from build123d import *

# Parameters (mm, degrees)
DOME_TRIM_SKETCH_W           = 13.999999999999993
DOME_TRIM_SKETCH_H           = 5.000000000000014
DOME_TRIM_DEPTH              = 14
RETAINER_FEATURE_3_PROFILE_R = 3.0000000000000027
RETAINER_FEATURE_3_DEPTH     = 3
RETAINER_FEATURE_4_PROFILE_R = 3.0000000000000027
RETAINER_FEATURE_4_DEPTH     = 3
RETAINER_FEATURE_6_PROFILE_R = 1.1000000000000036
RETAINER_FEATURE_6_DEPTH     = 4.25
RETAINER_FEATURE_7_PROFILE_R = 2.1000000000000045
RETAINER_FEATURE_7_DEPTH     = 1.45
RETAINER_FEATURE_8_PROFILE_R = 1.1000000000000036
RETAINER_FEATURE_8_DEPTH     = 4.25
RETAINER_FEATURE_9_PROFILE_R = 2.1000000000000045
RETAINER_FEATURE_9_DEPTH     = 1.45
RETAINER_FEATURE_12_DEPTH    = 10


with BuildPart() as part:
    # Retainer Dome Sketch → Retainer Dome (revolve)
    with BuildSketch(Plane(origin=(0, -73, 0), x_dir=(-1, 0, 0), z_dir=(0, -1, 0))):
        with BuildLine():
            Line((76.48780366869515, -22.98076211353316), (66.09549882328189, -28.980762113533164))
            ThreePointArc((66.09549882328189, -28.980762113533164), (74.29165124598852, -31.176914536239792), (76.48780366869515, -22.98076211353316))
        make_face()
    revolve(axis=Axis((-62.63139720814413, -73, 30.98076211353316), (-0.8660254037844387, 0, -0.49999999999999994)))

    # Dome Trim Sketch → Dome Trim (cut)
    with BuildSketch(Plane(origin=(-36.156560608000376, 0, -20.874999999999996), x_dir=(-0.49999999999999944, 0, 0.866025403784439), z_dir=(-0.866025403784439, 0, -0.49999999999999944))):
        with Locations((58.145825622994224, -68.5)):
            Rectangle(DOME_TRIM_SKETCH_W, DOME_TRIM_SKETCH_H)
    extrude(amount=DOME_TRIM_DEPTH, mode=Mode.SUBTRACT)

    # Retainer Feature 3 profile → Retainer Feature 3 (add)
    with BuildSketch(Plane(origin=(0, -71.00000000000001, 0), x_dir=(-1, 0, 0), z_dir=(0, -1, 0))):
        with Locations((63.93043531382078, -30.23076211353316)):
            Circle(RETAINER_FEATURE_3_PROFILE_R)
    extrude(amount=RETAINER_FEATURE_3_DEPTH)

    # Retainer Feature 4 profile → Retainer Feature 4 (add)
    with BuildSketch(Plane(origin=(0, -71.00000000000001, 0), x_dir=(-1, 0, 0), z_dir=(0, -1, 0))):
        with Locations((78.65286717815624, -21.73076211353316)):
            Circle(RETAINER_FEATURE_4_PROFILE_R)
    extrude(amount=RETAINER_FEATURE_4_DEPTH)

    # Spherical Seat Sketch → Spherical Seat (revolve, cut)
    with BuildSketch(Plane(origin=(0, -73, 0), x_dir=(-1, 0, 0), z_dir=(0, -1, 0))):
        with BuildLine():
            Line((74.0196312679095, -24.405762113533164), (68.56367122406753, -27.55576211353316))
            ThreePointArc((68.56367122406753, -27.55576211353316), (72.86665124598852, -28.708742135454145), (74.0196312679095, -24.405762113533164))
        make_face()
    revolve(axis=Axis((-62.63139720814413, -73, 30.98076211353316), (-0.8660254037844387, 0, -0.49999999999999994)), mode=Mode.SUBTRACT)

    # Retainer Feature 6 profile → Retainer Feature 6 (cut)
    with BuildSketch(Plane(origin=(0, -70, 0), x_dir=(-1, 0, 0), z_dir=(0, -1, 0))):
        with Locations(Location((63.93043531382078, -30.23076211353316, 0), (0, 0, 270))):
            Circle(RETAINER_FEATURE_6_PROFILE_R)
    extrude(amount=RETAINER_FEATURE_6_DEPTH, mode=Mode.SUBTRACT)

    # Retainer Feature 7 profile → Retainer Feature 7 (cut)
    with BuildSketch(Plane(origin=(0, -72.8, 0), x_dir=(-1, 0, 0), z_dir=(0, -1, 0))):
        with Locations(Location((63.93043531382078, -30.23076211353316, 0), (0, 0, 90))):
            Circle(RETAINER_FEATURE_7_PROFILE_R)
    extrude(amount=RETAINER_FEATURE_7_DEPTH, mode=Mode.SUBTRACT)

    # Retainer Feature 8 profile → Retainer Feature 8 (cut)
    with BuildSketch(Plane(origin=(0, -70, 0), x_dir=(-1, 0, 0), z_dir=(0, -1, 0))):
        with Locations(Location((78.65286717815624, -21.73076211353316, 0), (0, 0, 270))):
            Circle(RETAINER_FEATURE_8_PROFILE_R)
    extrude(amount=RETAINER_FEATURE_8_DEPTH, mode=Mode.SUBTRACT)

    # Retainer Feature 9 profile → Retainer Feature 9 (cut)
    with BuildSketch(Plane(origin=(0, -72.8, 0), x_dir=(-1, 0, 0), z_dir=(0, -1, 0))):
        with Locations(Location((78.65286717815624, -21.73076211353316, 0), (0, 0, 90))):
            Circle(RETAINER_FEATURE_9_PROFILE_R)
    extrude(amount=RETAINER_FEATURE_9_DEPTH, mode=Mode.SUBTRACT)

    # Middle Right Fixed Compression Ball Reta → Retainer Feature 12 (cut)
    with BuildSketch(Plane(origin=(-14.254693004611807, 11.570307263062045, 11.176575862570404), x_dir=(-0.403732922701292, 0.3277035826977628, -0.854172165909264), z_dir=(0.6631997284167646, -0.5383086561091629, -0.5199902989343905))):
        Polygon((-14.819319931758496, -98.86212155097724), (-20.944840012243684, -100.71630701731351), (-19.843917391606514, -104.3533345651016), (-13.718397311121315, -102.49914909876533), align=None)
    extrude(amount=RETAINER_FEATURE_12_DEPTH, mode=Mode.SUBTRACT)


with BuildPart() as body_2:
    # Mirror1: mirrored copy
    add(part.part.mirror(Plane(origin=(0, 0, 0), x_dir=(0, 0, 1), z_dir=(0, -1, 0))))


solid = body_2.part
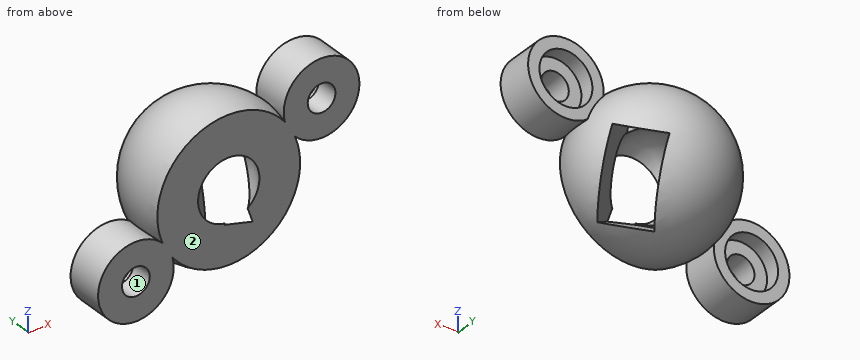
For this review, take the finished solid that the model builds, in its own axes (mm). Face numbers are marked on the shaded views. Round coordinates to 2 decimals unless told otherwise and drop trailing zeros. Write each loop counter-clockwise with the first axis right and the second up, starting at its lowest first coordinate (ties: lowest second). Pieces come first, ordered by that corner, then holes. Notation, with made-up numbers: (65, 22) -> (124, 22) arc R11 ccw to (124, 42) -> close; hole circle Ø7 at (50.25, -26). An arc over 180 degrees is marked (long way). Use CSV: the item, a comma, the result in double quotes.
(1) Consider section C-C, the plane z = 30.75. Give the boundary of the cut face in (x, y).
Computed values:
outline,"(-74.33, 71) -> (-68.25, 71) arc R3.64 ccw (long way) to start; (-66.89, 71) -> (-64.9, 71) -> (-64.9, 72.8) -> (-65.97, 72.8) -> (-65.97, 74) -> (-66.89, 74) -> close; (-62.96, 71) -> (-60.98, 71) -> (-60.98, 74) -> (-61.9, 74) -> (-61.9, 72.8) -> (-62.96, 72.8) -> close"
(2) Draft analysis for pull direction X (two halves, no side actions). For the marked faces 1 and 2, state which applies: +X half, -X half, draft (parallel to the pull), parting line (faces both ways), or undercut.
Computed values:
face 1,"undercut"
face 2,"draft"
(3) Consider section B-B, the plane y = 71.5. Give the boundary of the cut face in (x, z), plus the area to 3 significant figures.
Computed values:
outline,"(-76.78, 24.07) arc R3 ccw (long way) to (-75.69, 22.18) arc R5.81 ccw to (-65.8, 27.89) arc R3 ccw (long way) to (-66.9, 29.78) arc R5.81 ccw to start; hole circle Ø2.2 at (-78.65, 21.73); hole (-72.19, 23.28) -> (-68.78, 22.43) -> (-69.33, 24.02) arc R2.77 ccw (long way) to (-72.14, 23.34) -> close; hole circle Ø2.2 at (-63.93, 30.23)"
area,"128 mm²"
(4) Consider section D-D, the plane z = 28.75. Give the boundary of the cut face in (x, y).
Computed values:
outline,"(-76.22, 71) -> (-61.32, 71) -> (-61.32, 74) -> (-62.44, 74) -> (-62.44, 72.8) -> (-65.42, 72.8) -> (-65.42, 74) -> (-66.06, 74) arc R5.32 ccw (long way) to start; hole circle Ø3 at (-71.29, 73); hole (-70.19, 74.32) -> (-69.35, 73.28) -> (-68.87, 73.82) -> close"
(5) Consider section A-A, the plane x = -78.25. Give the boundary of the cut face in (y, z).
Computed values:
outline,"(71, 18.76) -> (74, 18.76) -> (74, 19.67) -> (72.8, 19.67) -> (72.8, 20.71) -> (71, 20.71) -> close; (71, 22.75) -> (72.8, 22.75) -> (72.8, 23.79) -> (74, 23.79) -> (74, 24.7) -> (71, 24.7) -> close"
(6) To check wall thickness, follow L1, parallel to X at y = 73.75, z = 31; L2, parallel to Z at x = -78.5, y = 73.75; L3, parallel to X at y = 72.75, z = 26.75. State the ranges of each line that lie inside material, in increasing order. Write a range as [from, to].
Computed values:
L1,"[-74.49, -68.09], [-66.83, -65.88], [-61.98, -61.03]"
L2,"[18.73, 19.64], [23.83, 24.73]"
L3,"[-77.24, -74.34], [-68.25, -65.35]"
(7) Clearance check with flat-ended pins moving along their axes: P1, Ø2, axis at x = -66.5, y = 77, coming from the +Z side; P2, Ø7.5, axis at x = -68, z = 29, coming from the -Y side; P3, Ø6.5, axis at x = -78.65, z = 21.73, coming from the +Y side; P4, Ø6, axis at y = 75.5, z = 30, coming from the +X side. State where each tip first meets the part, or that it passes through.
Computed values:
P1,"z = 28.9"
P2,"y = 71"
P3,"y = 75.91"
P4,"x = -60.93"
